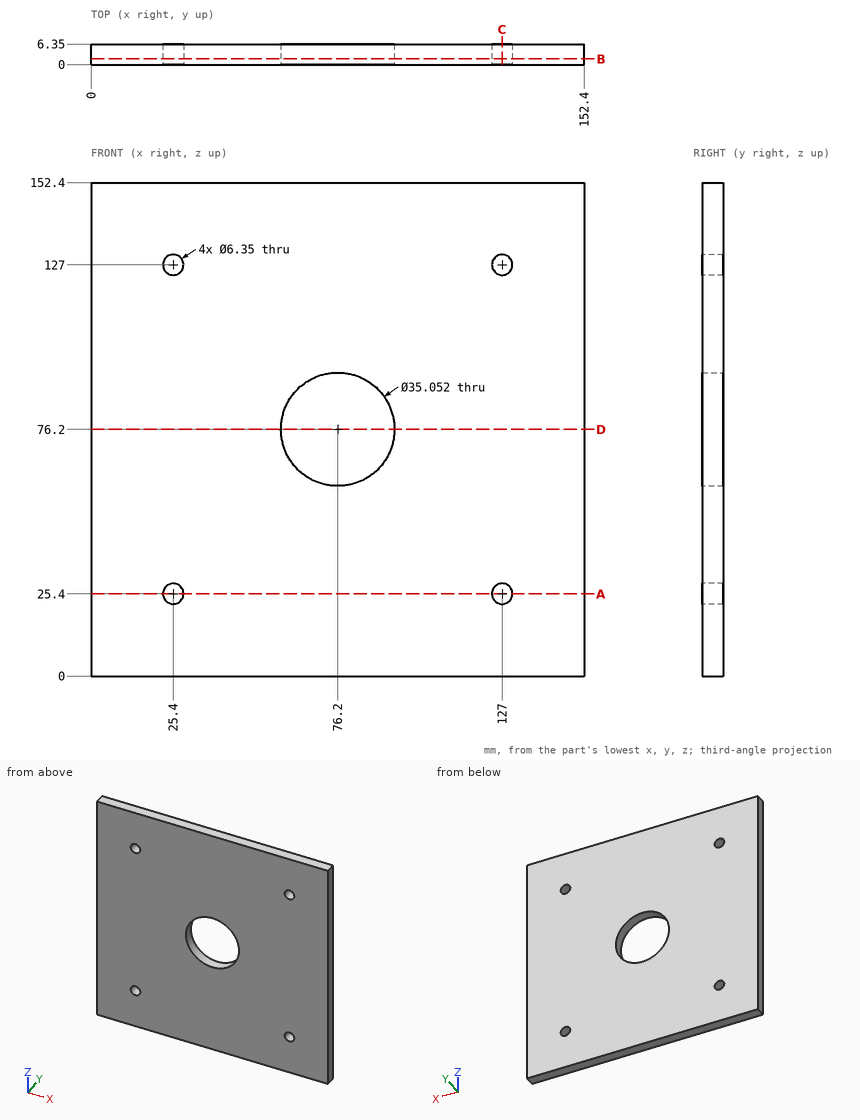
Geometry: see drawing. Coordinates: mm, zero at the bounding-box minimum. Give positions to 0.01 mm unless a question says otherwise; leave off trailing zeros. Write each loop counter-clockwise with the first axis right and the second up, starting at its lowest first coordinate (ties: lowest second). Pieces come first, ordered by that corner, then holes. Notation, with made-up numbers: M -33,43.25 L -3,43.25 A26 ccw -3,58.25 Z; hole C -16,-38.5 d2. An arc over 180 degrees is marked long. Answer in a Markdown table with one row per item. Add a question column.
(1) Section A-A on z = 25.4. Return loops of the section in (x, y) (3 decimals), and give its area (3 significant figures).
(2) Section C-C on x = 127. Return loops of the section in (y, z) (3 decimals).
(3) Section B-B on y = 1.75. Return loops of the section in (x, z) (3 decimals).
(4) Ray query, line 1 (X direction, y = 3.5, z = 127) (3 decimals); line 2 (X direction, y = 1.5, z = 76.2); line 3 (X direction, y = 1.75, z = 125). Return the intervals inside material, ascending.
(5) Section D-D on z = 76.2. Return loops of the section in (x, y), and give its area (3 significant figures).
Result set:
| question | item | result |
|---|---|---|
| 1 | outline | M 0,0 L 22.225,0 L 22.225,6.35 L 0,6.35 Z; M 28.575,0 L 123.825,0 L 123.825,6.35 L 28.575,6.35 Z; M 130.175,0 L 152.4,0 L 152.4,6.35 L 130.175,6.35 Z |
| 1 | area | 887 mm^2 |
| 2 | outline | M 0,0 L 6.35,0 L 6.35,22.225 L 0,22.225 Z; M 0,28.575 L 6.35,28.575 L 6.35,123.825 L 0,123.825 Z; M 0,130.175 L 6.35,130.175 L 6.35,152.4 L 0,152.4 Z |
| 3 | outline | M 0,0 L 152.4,0 L 152.4,152.4 L 0,152.4 Z; hole C 25.4,25.4 d6.35; hole C 25.4,127 d6.35; hole C 76.2,76.2 d35.052; hole C 127,25.4 d6.35; hole C 127,127 d6.35 |
| 4 | line 1 | x = 0 to 22.225, 28.575 to 123.825, 130.175 to 152.4 |
| 4 | line 2 | x = 0 to 58.67, 93.73 to 152.4 |
| 4 | line 3 | x = 0 to 22.93, 27.87 to 124.53, 129.47 to 152.4 |
| 5 | outline | M 0,0 L 58.67,0 L 58.67,6.35 L 0,6.35 Z; M 93.73,0 L 152.4,0 L 152.4,6.35 L 93.73,6.35 Z |
| 5 | area | 745 mm^2 |
